```python
from build123d import *

# Parameters (mm, degrees)
F1_DEPTH = 2.5
F3_R     = 10
F4_D     = 4
F5_R     = 1
F6_DEPTH = 6
F7_R     = 1.5
F8_DEPTH = 7


with BuildPart() as f1:
    # F0 (on Top) → F1 (new body)
    with BuildSketch(Plane.XY):
        with BuildLine():
            ThreePointArc((20, -2.5), (21.767766953, -1.767766953), (22.5, 0))
            ThreePointArc((22.5, 0), (21.767766953, 1.767766953), (20, 2.5))
            ThreePointArc((20, 2.5), (18.232233047, 1.767766953), (17.5, 0))
            ThreePointArc((17.5, 0), (18.232233047, -1.767766953), (20, -2.5))
        make_face()
        with BuildLine():
            ThreePointArc((17.5, 0), (18.232233047, 1.767766953), (20, 2.5))
            Line((20, 2.5), (1.443375673, 2.5))
            Line((1.443375673, 2.5), (2.1650635095, 1.25))
            ThreePointArc((2.1650635095, 1.25), (2.4148145657, 0.6470476128), (2.5, 0))
            Line((2.5, 0), (17.5, 0))
        make_face()
        with BuildLine():
            Line((1.443375673, -2.5), (20, -2.5))
            ThreePointArc((20, -2.5), (18.232233047, -1.767766953), (17.5, 0))
            Line((17.5, 0), (2.5, 0))
            ThreePointArc((2.5, 0), (2.4148145657, -0.6470476128), (2.1650635095, -1.25))
            Line((2.1650635095, -1.25), (1.443375673, -2.5))
        make_face()
        with BuildLine():
            Line((2.1650635095, 1.25), (1.443375673, 2.5))
            Line((1.443375673, 2.5), (0, 2.5))
            ThreePointArc((0, 2.5), (1.25, 2.1650635095), (2.1650635095, 1.25))
        make_face()
        with BuildLine():
            Line((0, 2.5), (1.443375673, 2.5))
            Line((1.443375673, 2.5), (-7.8349364905, 18.5705080757))
            ThreePointArc((-7.8349364905, 18.5705080757), (-7.5851854343, 17.9675556884), (-7.5, 17.3205080757))
            ThreePointArc((-7.5, 17.3205080757), (-7.8349364905, 16.0705080757), (-8.75, 15.1554445662))
            Line((-8.75, 15.1554445662), (-1.25, 2.1650635095))
            ThreePointArc((-1.25, 2.1650635095), (-0.6470476128, 2.4148145657), (0, 2.5))
        make_face()
        with BuildLine():
            Line((-7.8349364905, -18.5705080757), (1.443375673, -2.5))
            Line((1.443375673, -2.5), (0, -2.5))
            ThreePointArc((0, -2.5), (-0.6470476128, -2.4148145657), (-1.25, -2.1650635095))
            Line((-1.25, -2.1650635095), (-8.75, -15.1554445662))
            ThreePointArc((-8.75, -15.1554445662), (-7.8349364905, -16.0705080757), (-7.5, -17.3205080757))
            ThreePointArc((-7.5, -17.3205080757), (-7.5851854343, -17.9675556884), (-7.8349364905, -18.5705080757))
        make_face()
        with BuildLine():
            Line((0, -2.5), (1.443375673, -2.5))
            Line((1.443375673, -2.5), (2.1650635095, -1.25))
            ThreePointArc((2.1650635095, -1.25), (1.25, -2.1650635095), (0, -2.5))
        make_face()
        with BuildLine():
            ThreePointArc((-7.5, 17.3205080757), (-7.5851854343, 17.9675556884), (-7.8349364905, 18.5705080757))
            ThreePointArc((-7.8349364905, 18.5705080757), (-11.25, 19.4855715851), (-12.1650635095, 16.0705080757))
            ThreePointArc((-12.1650635095, 16.0705080757), (-10.6470476128, 14.90569351), (-8.75, 15.1554445662))
            ThreePointArc((-8.75, 15.1554445662), (-7.8349364905, 16.0705080757), (-7.5, 17.3205080757))
        make_face()
        with BuildLine():
            ThreePointArc((-12.1650635095, -16.0705080757), (-11.25, -19.4855715851), (-7.8349364905, -18.5705080757))
            ThreePointArc((-7.8349364905, -18.5705080757), (-7.5851854343, -17.9675556884), (-7.5, -17.3205080757))
            ThreePointArc((-7.5, -17.3205080757), (-7.8349364905, -16.0705080757), (-8.75, -15.1554445662))
            ThreePointArc((-8.75, -15.1554445662), (-10.6470476128, -14.90569351), (-12.1650635095, -16.0705080757))
        make_face()
        with BuildLine():
            ThreePointArc((-2.1650635095, 1.25), (-1.767766953, 1.767766953), (-1.25, 2.1650635095))
            Line((-1.25, 2.1650635095), (-8.75, 15.1554445662))
            ThreePointArc((-8.75, 15.1554445662), (-10.6470476128, 14.90569351), (-12.1650635095, 16.0705080757))
            Line((-12.1650635095, 16.0705080757), (-2.8867513459, 0))
            Line((-2.8867513459, 0), (-2.1650635095, 1.25))
        make_face()
        with BuildLine():
            Line((-8.75, -15.1554445662), (-1.25, -2.1650635095))
            ThreePointArc((-1.25, -2.1650635095), (-1.767766953, -1.767766953), (-2.1650635095, -1.25))
            Line((-2.1650635095, -1.25), (-2.8867513459, 0))
            Line((-2.8867513459, 0), (-12.1650635095, -16.0705080757))
            ThreePointArc((-12.1650635095, -16.0705080757), (-10.6470476128, -14.90569351), (-8.75, -15.1554445662))
        make_face()
        with BuildLine():
            ThreePointArc((-2.1650635095, -1.25), (-2.5, 0), (-2.1650635095, 1.25))
            Line((-2.1650635095, 1.25), (-2.8867513459, 0))
            Line((-2.8867513459, 0), (-2.1650635095, -1.25))
        make_face()
        with BuildLine():
            Line((-1.25, -2.1650635095), (0, 0))
            Line((0, 0), (-1.25, 2.1650635095))
            ThreePointArc((-1.25, 2.1650635095), (-1.767766953, 1.767766953), (-2.1650635095, 1.25))
            ThreePointArc((-2.1650635095, 1.25), (-2.5, 0), (-2.1650635095, -1.25))
            ThreePointArc((-2.1650635095, -1.25), (-1.767766953, -1.767766953), (-1.25, -2.1650635095))
        make_face()
        with BuildLine():
            Line((0, 0), (2.5, 0))
            ThreePointArc((2.5, 0), (2.4148145657, 0.6470476128), (2.1650635095, 1.25))
            ThreePointArc((2.1650635095, 1.25), (1.25, 2.1650635095), (0, 2.5))
            ThreePointArc((0, 2.5), (-0.6470476128, 2.4148145657), (-1.25, 2.1650635095))
            Line((-1.25, 2.1650635095), (0, 0))
        make_face()
        with BuildLine():
            ThreePointArc((2.1650635095, -1.25), (2.4148145657, -0.6470476128), (2.5, 0))
            Line((2.5, 0), (0, 0))
            Line((0, 0), (-1.25, -2.1650635095))
            ThreePointArc((-1.25, -2.1650635095), (-0.6470476128, -2.4148145657), (0, -2.5))
            ThreePointArc((0, -2.5), (1.25, -2.1650635095), (2.1650635095, -1.25))
        make_face()
    extrude(amount=F1_DEPTH)

    # F3
    f3_edges = [f1.edges().sort_by_distance(p)[0] for p in [
        (1.443376, -2.5, 1.25),
        (-2.886751, 0, 1.25),
        (1.443376, 2.5, 1.25),
    ]]
    fillet(f3_edges, radius=F3_R)

    # F4 (through all)
    with Locations(Plane(origin=(0, 0, 0), x_dir=(1, 0, 0), z_dir=(0, 0, -1))):
        with Locations((0, 0)):
            Hole(F4_D / 2)

    # F5 (on Top) → F6 (join)
    with BuildSketch(Plane.XY):
        with Locations((-1.9745181319, -3.478689142)):
            Circle(F5_R)
    extrude(amount=F6_DEPTH)

    # F7 (on Top) → F8 (cut)
    with BuildSketch(Plane.XY):
        with Locations((4, 0)):
            Circle(F7_R)
    extrude(amount=F8_DEPTH, mode=Mode.SUBTRACT)


solid = f1.part
```
Verification items for the finished model (mm, model axes). A direction names the side the tool comes from. Give positions to 0.01 mm unless a question says otherwise; leave off trailing zeros. Order: outer loops, then holes, each group sorted by start corner. A loop starts at its lowest first (then second) coordinate and runs counter-clockwise, first axis right, second up. Notation, with made-up numbers: (-5, -26.5) -> (34, -26.5) arc R31 cw to (34, 4.5) -> close; hole circle Ø7 at (0.25, 83). An arc over 180 degrees is marked (long way). Use a Markdown table: item, result.
1) Mould release check, pull along Y, two halves, no side actions. Record for faces 1 (the flat face through (-9.014, 10.613, 1.232)), 2 (the cylindrical face through (-2.71, -2.8, 4.23)), 3 (the flat face through (-2, -1, 2.5)): pulls with the +Y half, pulls with the -Y half, needs draft (parallel to the pull), parting line crosses it, or undercut.
Results:
| item | result |
|---|---|
| face 1 | undercut |
| face 2 | parting line crosses it |
| face 3 | needs draft |
2) Material ranges on probe 1 along Z at (x, y) = (-4, 10.5); probe 2 along Y at (x, z) = (0, 1.75); probe 3 along Y at (x, z) = (9.5, 1.1), recorded low to high.
Results:
| item | result |
|---|---|
| probe 1 | 0 to 2.5 |
| probe 2 | -5.58 to -2, 2 to 5.58 |
| probe 3 | -2.5 to 2.5 |
3) Section check C-C, the plane z = 1.85. Record the boundary of the cut face in (x, y).
Results:
| item | result |
|---|---|
| outline | (-12.17, -16.07) arc R2.5 ccw to (-7.83, -18.57) -> (-1.44, -7.5) arc R10 cw to (7.22, -2.5) -> (20, -2.5) arc R2.5 ccw to (20, 2.5) -> (7.22, 2.5) arc R10 cw to (-1.44, 7.5) -> (-7.83, 18.57) arc R2.5 ccw to (-12.17, 16.07) -> (-5.77, 5) arc R10 cw to (-5.77, -5) -> close; hole circle Ø4 at (0, 0); hole circle Ø3 at (4, 0) |
4) Depth check by flat-ended pin: pin 1 Ø1.5 at (y, z) = (-13.5, 4) entering from -X; pin 2 Ø1.2 at (x, z) = (16.5, 1.5) entering from -Y; pin 3 Ø4 at (x, y) = (4, 0) entering from -Z; pin 4 Ø0.8 at (x, z) = (16.5, 1.5) entering from +Y. Enter the tip coordinate at first touch or a pass-through.
Results:
| item | result |
|---|---|
| pin 1 | through |
| pin 2 | y = -2.5 |
| pin 3 | z = 0 |
| pin 4 | y = 2.5 |
5) Section check D-D, the plane x = 1.5. Record the boundary of the cut face in (y, z).
Results:
| item | result |
|---|---|
| outline | (-4.3, 0) -> (-1.32, 0) -> (-1.32, 2.5) -> (-4.3, 2.5) -> close; (1.32, 0) -> (4.3, 0) -> (4.3, 2.5) -> (1.32, 2.5) -> close |
6) Section check A-A, the plane y = 1. Record the boundary of the cut face in (x, z).
Results:
| item | result |
|---|---|
| outline | (-4.48, 0) -> (-1.73, 0) -> (-1.73, 2.5) -> (-4.48, 2.5) -> close; (1.73, 0) -> (2.88, 0) -> (2.88, 2.5) -> (1.73, 2.5) -> close; (5.12, 0) -> (22.29, 0) -> (22.29, 2.5) -> (5.12, 2.5) -> close |
7) Tool access check on faces 4 (the flat face through (-8.925, -10.458, 1.232)), 5 (the flat face through (14, -2.5, 1)), 6 (the flat face through (14, 2.5, 1)). Record the directions out of +Z, -Z, +X, -X, +Y, -Y that give a thin tool (end or side, any length) a straight path to the whole face; none if there is none.
Results:
| item | result |
|---|---|
| face 4 | +Z, -Z, -X |
| face 5 | +Z, -Z, +X, -Y |
| face 6 | +Z, -Z, +X, +Y |
8) Section check B-B, the plane x = -9. Record the boundary of the cut face in (y, z).
Results:
| item | result |
|---|---|
| outline | (-19.61, 0) -> (-10.59, 0) -> (-10.59, 2.5) -> (-19.61, 2.5) -> close; (10.59, 0) -> (19.61, 0) -> (19.61, 2.5) -> (10.59, 2.5) -> close |
